The drawing under review shows one solid part. Ordinate dimensions are in mm from its lowest x, y, z. Round coordinates to 2 decimals unless told otherwise and drop trailing zeros. Order: outer loops, then holes, each group sorted by start corner. A loop starts at its lowest first (then second) coordinate and runs counter-clockwise, first axis right, second up.
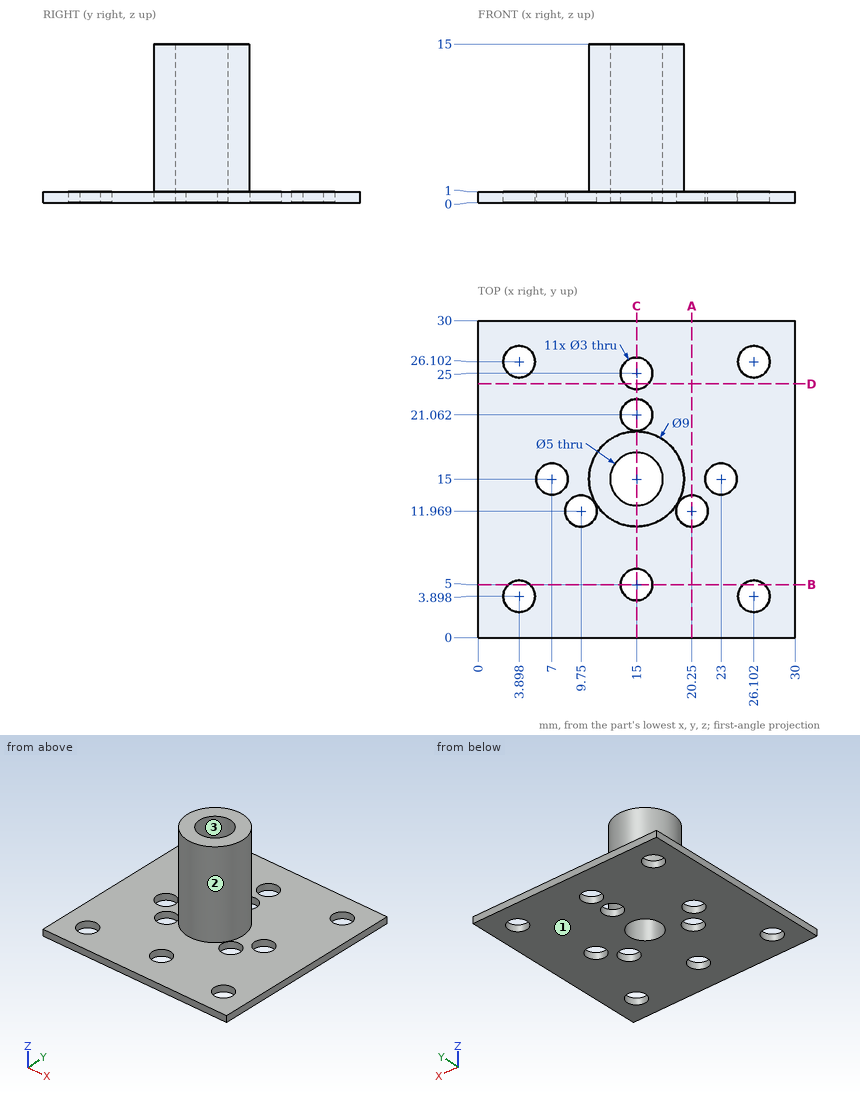
Q1. Take a section at D-D, the plane y = 24. State the section outline as (x, z) points.
Q2. Take a section at A-A, the plane x = 20.25. State the section outline as (y, z) points, plus the area to 3 significant figures.
Q3. Clearance check with flat-ended pins moving along their axes: pin 1 (3.5 mm diameter, centred on x = 3.9, y = 26.1, fed in from +Z); pin 2 (4 mm diameter, centred on x = 14, z = 13, fed in from +Y); pin 3 (6 mm diameter, centred on y = 9, z = 13.5, fed in from -X) (1 decimal). State where each tip first meets the part, or that it passes through.
Q4. Take a section at B-B, the plane y = 5. State the section outline as (x, z) points.
Q5. Wall thickness on line 1 (Y direction, x = 7, z = 0.3); line 2 (X direction, y = 5, z = 0.35) (1 decimal); line 3 (Z direction, x = 7.5, y = 24.25): over which ranges is each line inside the solid? List them lowest first.
Q6. Mouldability with a two-part tool opening along Y and no side actions: class the marked faces 1, 2 and 3 as +Y half, -Y half, draft (parallel to the pull), parting line (faces both ways), or undercut.
Q7. Take a section at C-C, the plane x = 15. State the section outline as (y, z) points.
Working result:
1. outline: (0, 0) - (13.88, 0) - (13.88, 1) - (0, 1) - close; (16.12, 0) - (30, 0) - (30, 1) - (16.12, 1) - close
2. outline: (0, 0) - (10.47, 0) - (10.47, 1) - (0, 1) - close; (13.47, 0) - (30, 0) - (30, 1) - (13.47, 1) - close
2. area: 27.0 mm2
3. pin 1: stops at z = 1
3. pin 2: stops at y = 19.5
3. pin 3: stops at x = 11.6
4. outline: (0, 0) - (2.88, 0) - (2.88, 1) - (0, 1) - close; (4.92, 0) - (13.5, 0) - (13.5, 1) - (4.92, 1) - close; (16.5, 0) - (25.08, 0) - (25.08, 1) - (16.5, 1) - close; (27.12, 0) - (30, 0) - (30, 1) - (27.12, 1) - close
5. line 1: y = 0 to 13.5, 16.5 to 30
5. line 2: x = 0 to 2.9, 4.9 to 13.5, 16.5 to 25.1, 27.1 to 30
5. line 3: z = 0 to 1
6. face 1: draft
6. face 2: parting line
6. face 3: undercut
7. outline: (0, 0) - (3.5, 0) - (3.5, 1) - (0, 1) - close; (6.5, 0) - (12.5, 0) - (12.5, 15) - (10.5, 15) - (10.5, 1) - (6.5, 1) - close; (17.5, 0) - (19.56, 0) - (19.56, 1) - (19.5, 1) - (19.5, 15) - (17.5, 15) - close; (22.56, 0) - (23.5, 0) - (23.5, 1) - (22.56, 1) - close; (26.5, 0) - (30, 0) - (30, 1) - (26.5, 1) - close
